Work out the finished part from the listing and answer in its coordinate system (mm). Round coordinates to 2 decimals unless told otherwise and drop trailing zeros.
1. Flat-ended cylindrical pins translate along their axes: pin 1 Ø3 at (x, z) = (2.5, 249.5) entering from -Y; pin 2 Ø1.9 at (x, z) = (-1.5, 201.5) entering from +Y; pin 3 Ø1.5 at (y, z) = (3.5, 112) entering from +X; pin 4 Ø2 at (x, y) = (7, 2) entering from -Z. Find the tip coordinate at first contact, or state that the pin passes through.
2. Find section A-A (z = 288). Count the separate pieces of the cut face and the enclosed holes in it, and give its area (3 significant figures).
3. Straight lines are drawn through the part: probe 1 along X at (y, z) = (4.25, 362); probe 2 along Y at (x, z) = (11, 276); probe 3 along Y at (x, z) = (11.5, 255). For each, find the intervals that lie inside material, in ascending order.
```python
from build123d import *

# Parameters (mm, degrees)
SKETCH_28_R     = 2.1
EXTRUDE_1_DEPTH = 400


with BuildPart() as part:
    # 草图28 → 凸台-拉伸1 (new body)
    with BuildSketch(Plane.XY):
        with BuildLine():
            Line((-5.5, 0), (-5.8, -0.519615242))
            Line((-5.8, -0.519615242), (-5.8, -4.385786438))
            Line((-5.8, -4.385786438), (-9.664213562, -8.25))
            Line((-9.664213562, -8.25), (-13.1, -8.25))
            Line((-13.1, -8.25), (-13.1, -4.1))
            Line((-13.1, -4.1), (-14.2, -4.1))
            Line((-14.2, -4.1), (-14.2, -5.1))
            Line((-14.2, -5.1), (-15, -5.1))
            Line((-15, -5.1), (-15, -13))
            ThreePointArc((-15, -13), (-14.414213562, -14.414213562), (-13, -15))
            Line((-13, -15), (-5.1, -15))
            Line((-5.1, -15), (-5.1, -14.2))
            Line((-5.1, -14.2), (-4.1, -14.2))
            Line((-4.1, -14.2), (-4.1, -13.1))
            Line((-4.1, -13.1), (-8.25, -13.1))
            Line((-8.25, -13.1), (-8.25, -9.664213562))
            Line((-8.25, -9.664213562), (-4.385786438, -5.8))
            Line((-4.385786438, -5.8), (-0.519615242, -5.8))
            Line((-0.519615242, -5.8), (0, -5.5))
            Line((0, -5.5), (0.519615242, -5.8))
            Line((0.519615242, -5.8), (4.385786438, -5.8))
            Line((4.385786438, -5.8), (8.25, -9.664213562))
            Line((8.25, -9.664213562), (8.25, -13.1))
            Line((8.25, -13.1), (4.1, -13.1))
            Line((4.1, -13.1), (4.1, -14.2))
            Line((4.1, -14.2), (5.1, -14.2))
            Line((5.1, -14.2), (5.1, -15))
            Line((5.1, -15), (13, -15))
            ThreePointArc((13, -15), (14.414213562, -14.414213562), (15, -13))
            Line((15, -13), (15, -5.1))
            Line((15, -5.1), (14.2, -5.1))
            Line((14.2, -5.1), (14.2, -4.1))
            Line((14.2, -4.1), (13.1, -4.1))
            Line((13.1, -4.1), (13.1, -8.25))
            Line((13.1, -8.25), (9.664213562, -8.25))
            Line((9.664213562, -8.25), (5.8, -4.385786438))
            Line((5.8, -4.385786438), (5.8, -0.519615242))
            Line((5.8, -0.519615242), (5.5, 0))
            Line((5.5, 0), (5.8, 0.519615242))
            Line((5.8, 0.519615242), (5.8, 4.385786438))
            Line((5.8, 4.385786438), (9.664213562, 8.25))
            Line((9.664213562, 8.25), (13.1, 8.25))
            Line((13.1, 8.25), (13.1, 4.1))
            Line((13.1, 4.1), (14.2, 4.1))
            Line((14.2, 4.1), (14.2, 5.1))
            Line((14.2, 5.1), (15, 5.1))
            Line((15, 5.1), (15, 13))
            ThreePointArc((15, 13), (14.414213562, 14.414213562), (13, 15))
            Line((13, 15), (5.1, 15))
            Line((5.1, 15), (5.1, 14.2))
            Line((5.1, 14.2), (4.1, 14.2))
            Line((4.1, 14.2), (4.1, 13.1))
            Line((4.1, 13.1), (8.25, 13.1))
            Line((8.25, 13.1), (8.25, 9.664213562))
            Line((8.25, 9.664213562), (4.385786438, 5.8))
            Line((4.385786438, 5.8), (0.519615242, 5.8))
            Line((0.519615242, 5.8), (0, 5.5))
            Line((0, 5.5), (-0.519615242, 5.8))
            Line((-0.519615242, 5.8), (-4.385786438, 5.8))
            Line((-4.385786438, 5.8), (-8.25, 9.664213562))
            Line((-8.25, 9.664213562), (-8.25, 13.1))
            Line((-8.25, 13.1), (-4.1, 13.1))
            Line((-4.1, 13.1), (-4.1, 14.2))
            Line((-4.1, 14.2), (-5.1, 14.2))
            Line((-5.1, 14.2), (-5.1, 15))
            Line((-5.1, 15), (-13, 15))
            ThreePointArc((-13, 15), (-14.414213562, 14.414213562), (-15, 13))
            Line((-15, 13), (-15, 5.1))
            Line((-15, 5.1), (-14.2, 5.1))
            Line((-14.2, 5.1), (-14.2, 4.1))
            Line((-14.2, 4.1), (-13.1, 4.1))
            Line((-13.1, 4.1), (-13.1, 8.25))
            Line((-13.1, 8.25), (-9.664213562, 8.25))
            Line((-9.664213562, 8.25), (-5.8, 4.385786438))
            Line((-5.8, 4.385786438), (-5.8, 0.519615242))
            Line((-5.8, 0.519615242), (-5.5, 0))
        make_face()
        with Locations((11.5, -11.5)):
            Circle(SKETCH_28_R, mode=Mode.SUBTRACT)
        with Locations((-11.5, -11.5)):
            Circle(SKETCH_28_R, mode=Mode.SUBTRACT)
        with Locations((11.5, 11.5)):
            Circle(SKETCH_28_R, mode=Mode.SUBTRACT)
        with Locations((-11.5, 11.5)):
            Circle(SKETCH_28_R, mode=Mode.SUBTRACT)
        with BuildLine():
            Line((2.474873733, -3.535533907), (1.814611277, -2.875271451))
            ThreePointArc((1.814611277, -2.875271451), (0, -3.400000001), (-1.814611277, -2.875271452))
            Line((-1.814611277, -2.875271452), (-2.47487373, -3.535533905))
            ThreePointArc((-2.47487373, -3.535533905), (-3.535533904, -3.535533907), (-3.535533905, -2.474873733))
            Line((-3.535533905, -2.474873733), (-2.875271451, -1.814611279))
            ThreePointArc((-2.875271451, -1.814611279), (-3.400000001, 0), (-2.87527145, 1.814611278))
            Line((-2.87527145, 1.814611278), (-3.535533908, 2.474873736))
            ThreePointArc((-3.535533908, 2.474873736), (-3.535533907, 3.535533907), (-2.474873737, 3.535533906))
            Line((-2.474873737, 3.535533906), (-1.814611279, 2.875271449))
            ThreePointArc((-1.814611279, 2.875271449), (-1e-09, 3.399999999), (1.814611277, 2.875271449))
            Line((1.814611277, 2.875271449), (2.474873733, 3.535533905))
            ThreePointArc((2.474873733, 3.535533905), (3.535533905, 3.535533905), (3.535533905, 2.474873733))
            Line((3.535533905, 2.474873733), (2.875271449, 1.814611277))
            ThreePointArc((2.875271449, 1.814611277), (3.399999999, -1e-09), (2.875271449, -1.814611279))
            Line((2.875271449, -1.814611279), (3.535533905, -2.474873735))
            ThreePointArc((3.535533905, -2.474873735), (3.535533905, -3.535533907), (2.474873733, -3.535533907))
        make_face(mode=Mode.SUBTRACT)
    extrude(amount=EXTRUDE_1_DEPTH)


solid = part.part
```
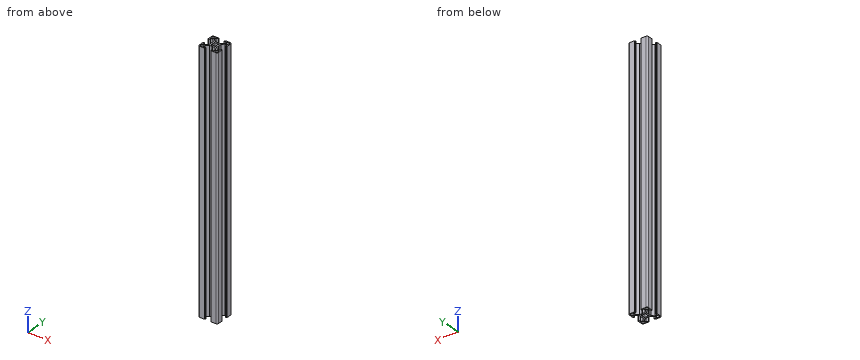
Worked answers:
1. pin 1: stops at y = -5.8
1. pin 2: stops at y = 5.8
1. pin 3: stops at x = 14.2
1. pin 4: passes through
2. separate pieces: 1
2. enclosed holes: 5
2. area: 305 mm2
3. probe 1: x = -14.2 to -13.1, -5.8 to 5.8, 13.1 to 14.2
3. probe 2: y = -15 to -13.54, -9.46 to -8.25, 8.25 to 9.46, 13.54 to 15
3. probe 3: y = -15 to -13.6, -9.4 to -8.25, 8.25 to 9.4, 13.6 to 15
